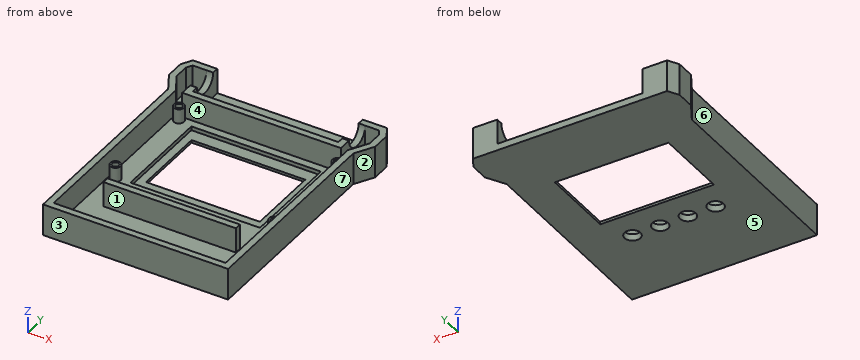
```python
from build123d import *

# Parameters (mm, degrees)
F2_DEPTH      = 12
F3_W          = 55
F3_H          = 15
F4_DEPTH      = 9.5
F6_DEPTH      = 9.5
F7_R          = 5
F8_DEPTH      = 57.5
F8_DEPTH_BACK = 2.5
F9_W          = 50
F9_H          = 2.5
F10_DEPTH     = 9.5
F11_W         = 43
F11_H         = 28
F11_R         = 3
F12_DEPTH     = 2.5
F13_W         = 49
F13_H         = 37.5
F14_DEPTH     = 1.5
F15_R         = 1.95
F16_DEPTH     = 5.5
F17_R         = 1.25
F18_DEPTH     = 6


with BuildPart() as f2:
    # F1 (on Top) → F2 (new body)
    with BuildSketch(Plane.XY):
        Polygon((-35, 38.5), (-35, -38.5), (35, -38.5), (35, 38.5), (39, 45.5), (39, 52.5), (36.6905989232, 56.5), (-36.6905989232, 56.5), (-39, 52.5), (-39, 45.5), align=None)
    extrude(amount=F2_DEPTH)

    # F3 (on face) → F4 (cut)
    with BuildSketch(Plane.XY.offset(12)):
        with Locations((0, 49)):
            Rectangle(F3_W, F3_H)
    extrude(amount=-F4_DEPTH, mode=Mode.SUBTRACT)

    # F5 (on face) → F6 (cut)
    with BuildSketch(Plane.XY.offset(12)):
        Polygon((-32.5, 39.1639110927), (-32.5, -36), (32.5, -36), (32.5, 39.1639110927), (36.5, 46.1639110927), (36.5, 51.8301270189), (35.2472232503, 54), (30, 54), (30, 39), (-30, 39), (-30, 54), (-35.2472232503, 54), (-36.5, 51.8301270189), (-36.5, 46.1639110927), align=None)
    extrude(amount=-F6_DEPTH, mode=Mode.SUBTRACT)

    # F7 (on face) → F8 (cut, two sides)
    with BuildSketch(Plane.YZ.offset(-27.5)) as f8_sk:
        with Locations((49, 12)):
            Circle(F7_R)
    extrude(amount=F8_DEPTH, mode=Mode.SUBTRACT)
    extrude(f8_sk.sketch, amount=-F8_DEPTH_BACK, mode=Mode.SUBTRACT)

    # F9 (on face) → F10 (join)
    with BuildSketch(Plane.XY.offset(2.5)):
        with Locations((0, -16.25)):
            Rectangle(F9_W, F9_H)
    extrude(amount=F10_DEPTH)

    # F11 (on face) → F12 (cut, through all)
    with BuildSketch(Plane.XY.offset(2.5)):
        with Locations((-0.22, 17.29)):
            Rectangle(F11_W, F11_H)
        with Locations((-15.72, -7.5)):
            Circle(F11_R)
        with Locations((-5.24, -7.5)):
            Circle(F11_R)
        with Locations((5.24, -7.5)):
            Circle(F11_R)
        with Locations((15.72, -7.5)):
            Circle(F11_R)
    extrude(amount=-F12_DEPTH, mode=Mode.SUBTRACT)

    # F13 (on face) → F14 (cut)
    with BuildSketch(Plane.XY.offset(2.5)):
        with Locations((-0.22, 17.29)):
            Rectangle(F13_W, F13_H)
    extrude(amount=-F14_DEPTH, mode=Mode.SUBTRACT)

    # F15 (on face) → F16 (join)
    with BuildSketch(Plane.XY.offset(2.5)):
        with Locations((-30, 37)):
            Circle(F15_R)
        with Locations((30, 37)):
            Circle(F15_R)
        with Locations((-30, -2)):
            Circle(F15_R)
        with Locations((30, -2)):
            Circle(F15_R)
    extrude(amount=F16_DEPTH)

    # F17 (on face) → F18 (cut)
    with BuildSketch(Plane.XY.offset(8)):
        with Locations((-30, 37)):
            Circle(F17_R)
        with Locations((30, 37)):
            Circle(F17_R)
        with Locations((30, -2)):
            Circle(F17_R)
        with Locations((-30, -2)):
            Circle(F17_R)
    extrude(amount=-F18_DEPTH, mode=Mode.SUBTRACT)


solid = f2.part
```
Could you check a few things on this model? Use its own coordinates, in mm. Face numbers are marked on the shaded views. A direction names the side the tool comes from. Round coordinates to 2 decimals unless told otherwise and drop trailing zeros. Order: outer loops, then holes, each group sorted by start corner. A loop starts at its lowest first (then second) coordinate and runs counter-clockwise, first axis right, second up. Notation, with made-up numbers: (2, 28.25) -> (40, 28.25) arc R26 cw to (40, 53.25) -> close; hole circle Ø10 at (37, 30.25). An arc over 180 degrees is marked (long way). One line per question, with ' | ' between items.
Q1. If we section it at A-A on y = -7.5: Write out the boundary of the cut face in (x, z), plus the area to 4 significant figures.
Computed values:
outline: (-35, 0) -> (-18.72, 0) -> (-18.72, 2.5) -> (-32.5, 2.5) -> (-32.5, 12) -> (-35, 12) -> close; (-12.72, 0) -> (-8.24, 0) -> (-8.24, 2.5) -> (-12.72, 2.5) -> close; (-2.24, 0) -> (2.24, 0) -> (2.24, 2.5) -> (-2.24, 2.5) -> close; (8.24, 0) -> (12.72, 0) -> (12.72, 2.5) -> (8.24, 2.5) -> close; (18.72, 0) -> (35, 0) -> (35, 12) -> (32.5, 12) -> (32.5, 2.5) -> (18.72, 2.5) -> close | area: 162.5 mm²
Q2. If I drill on line 1 (Y direction, x = 11.5, z = 4.5); line 2 (Y direction, x = -5.24, z = 1.5); line 3 (X direction, y = 21, z = 0.75), over which ranges is the centre line in solid material (lowest first)? Write a range as from..to.
Computed values:
line 1: -38.5..-36, -17.5..-15, 39..41.5 | line 2: -38.5..-10.5, -4.5..-1.46, 36.04..56.5 | line 3: -35..-21.72, 21.28..35
Q3. I'm going to push flat-ended pins straight in: pin 1 (4 mm diameter, centred on x = 30, y = 37, fed in from -Z); pin 2 (4 mm diameter, centred on y = -26.5, z = 6.5, fed in from +X); pin 3 (1.1 mm diameter, centred on y = 15.5, z = 0.5, fed in from -X); pin 4 (2 mm diameter, centred on x = 30, y = -2, fed in from +Z). Where does each tip first touch, or does it pass through?
Computed values:
pin 1: z = 0 | pin 2: x = 35 | pin 3: x = -35 | pin 4: z = 2
Q4. Which directions (+Z, -Z, +X, -X, +Y, -Y) give clear straight access to the entire face, cutting with the end or side of a thin tool? Please do the marked faces 4, 5, 6 and 7.
Computed values:
face 4: +Z | face 5: -Z, +X, -X, +Y, -Y | face 6: +Z, -Z, -X, -Y | face 7: +Z, -Z, +X, -Y
Q5. If we section it at B-B on x = -15.72: Write out the boundary of the cut face in (y, z).
Computed values:
outline: (-38.5, 0) -> (-10.5, 0) -> (-10.5, 2.5) -> (-15, 2.5) -> (-15, 12) -> (-17.5, 12) -> (-17.5, 2.5) -> (-36, 2.5) -> (-36, 12) -> (-38.5, 12) -> close; (-4.5, 0) -> (3.29, 0) -> (3.29, 1) -> (-1.46, 1) -> (-1.46, 2.5) -> (-4.5, 2.5) -> close; (31.29, 0) -> (56.5, 0) -> (56.5, 2.5) -> (41.5, 2.5) -> (41.5, 12) -> (39, 12) -> (39, 2.5) -> (36.04, 2.5) -> (36.04, 1) -> (31.29, 1) -> close
Q6. If we section it at C-C on y = 20.5: Write out the boundary of the cut face in (x, z).
Computed values:
outline: (-35, 0) -> (-21.72, 0) -> (-21.72, 1) -> (-24.72, 1) -> (-24.72, 2.5) -> (-32.5, 2.5) -> (-32.5, 12) -> (-35, 12) -> close; (21.28, 0) -> (35, 0) -> (35, 12) -> (32.5, 12) -> (32.5, 2.5) -> (24.28, 2.5) -> (24.28, 1) -> (21.28, 1) -> close
Q7. If we section it at D-D on y = 49: Write out the boundary of the cut face in (x, z).
Computed values:
outline: (-39, 0) -> (39, 0) -> (39, 12) -> (36.5, 12) -> (36.5, 2.5) -> (30, 2.5) -> (30, 7) -> (27.5, 7) -> (27.5, 2.5) -> (-27.5, 2.5) -> (-27.5, 7) -> (-30, 7) -> (-30, 2.5) -> (-36.5, 2.5) -> (-36.5, 12) -> (-39, 12) -> close
Q8. We'd pull the mould along X, two halves only. Please class the marked faces 1, 2 and 3: released by +X, released by -X, zero draft, split by the parting line, or undercut.
Computed values:
face 1: undercut | face 2: released by +X | face 3: zero draft
